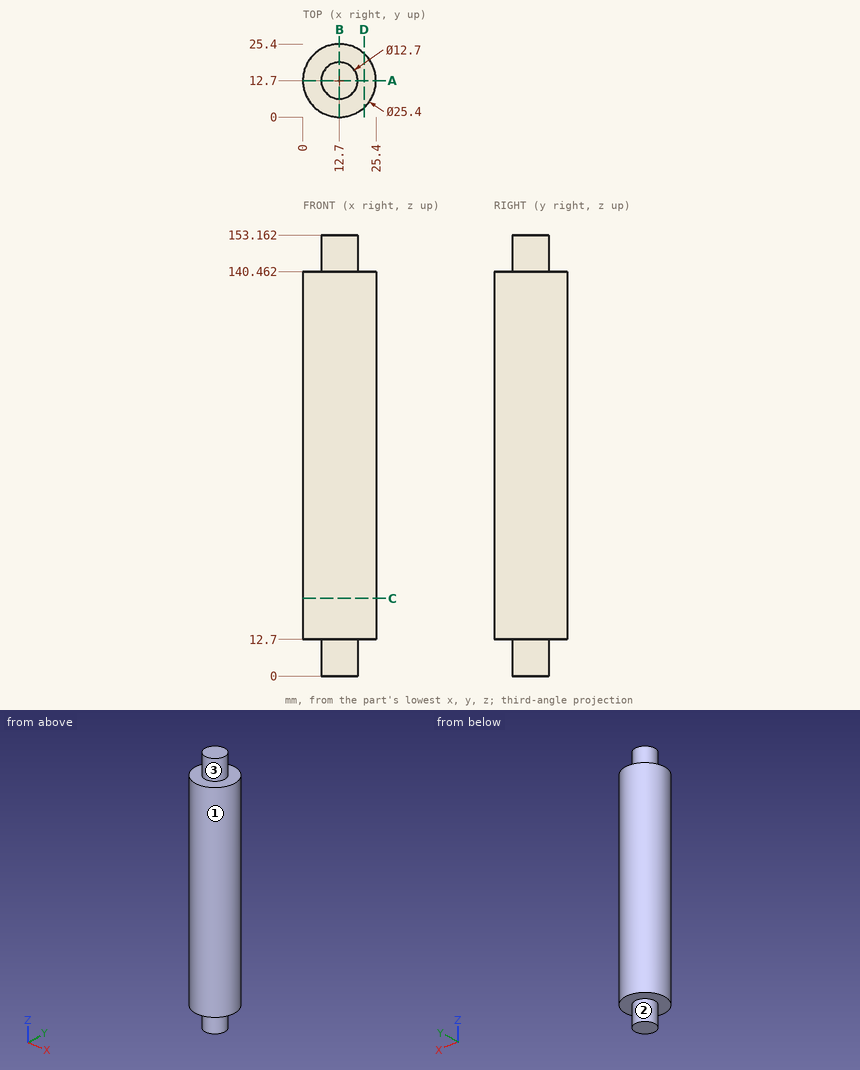
Geometry check sheet. Reference: drawing and pictorial views, mm from the part's lowest x, y, z. A direction names the side the tool comes from. Give positions to 0.01 mm unless a question says otherwise; leave off trailing zeros. Loops run counter-clockwise (first coordinate to the right, second up) from the corner with the lowest first, then second, coordinate; pieces in that order, holes last. Notation, with made-up numbers: M 34.25,77.25 L 53.25,77.25 A21 cw 53.25,87.25 Z; hole C 53.25,86.5 d8. An arc over 180 degrees is marked long. One line per question, with ' | ' between items.
Item 1: Section check A-A, the plane y = 12.7. Record the cut outline in (x, z), plus the area to 3 significant figures.
Completed:
outline: M 0,12.7 L 6.35,12.7 L 6.35,0 L 19.05,0 L 19.05,12.7 L 25.4,12.7 L 25.4,140.46 L 19.05,140.46 L 19.05,153.16 L 6.35,153.16 L 6.35,140.46 L 0,140.46 Z | area: 3,570 mm^2
Item 2: Thickness scan on line 1 (Z direction, x = 21.75, y = 13); line 2 (Y direction, x = 12, z = 67.5); line 3 (X direction, y = 17, z = 129). Record the ranges inside material, lowest first. Write a range as [from, to].
Completed:
line 1: z = [12.7, 140.46] | line 2: y = [0.02, 25.38] | line 3: x = [0.75, 24.65]
Item 3: Tool access check on the marked faces 1, 2 and 3. Record the directions out of +Z, -Z, +X, -X, +Y, -Y that give a thin tool (end or side, any length) a straight path to the whole face; none if there is none.
Completed:
face 1: +Z, -Z | face 2: -Z | face 3: +Z
Item 4: Depth check by flat-ended pin: P1, Ø12, axis at x = 8, z = 54.5, coming from the +Y side; P2, Ø4, axis at x = 6.5, z = 98.5, coming from the +Y side; P3, Ø1, axis at y = 7.5, z = 120.5, coming from the +X side; P4, Ø5, axis at y = 3.5, z = 15.5, coming from the -X side. Enter the tip coordinate at first touch or a pass-through.
Completed:
P1: stops at y = 25.4 | P2: stops at y = 24.69 | P3: stops at x = 24.5 | P4: stops at x = 1.91
Item 5: Section check C-C, the plane z = 27. Record the cut outline in (x, y), plus the area to 3 significant figures.
Completed:
outline: C 12.7,12.7 d25.4 | area: 507 mm^2
Item 6: Section check D-D, the plane x = 21.25. Record the cut outline in (y, z), plus the area to 3 significant figures.
Completed:
outline: M 3.31,12.7 L 22.09,12.7 L 22.09,140.46 L 3.31,140.46 Z | area: 2,400 mm^2
